Geometry check sheet. Reference: the model listing, model coordinates, mm. Give positions to 0.01 mm unless a question says otherwise; leave off trailing zeros. Loops run counter-clockwise (first coordinate to the right, second up) from the corner with the lowest first, then second, coordinate; pieces in that order, holes last. Notation, with made-up numbers: (84.25, 28.5) - (122.25, 28.5) arc R23 ccw to (122.25, 53.5) - close; hole circle Ø10 at (49.25, 28). An arc over 180 degrees is marked (long way). Use a Markdown table: item, result. Add a question column.
1. Cross-section at C-C on x = -27.35. Enter the section's corners in (y, z).
2. Material ranges on L1, parallel to Y at x = -61.55, z = 2.5; L2, parallel to X at y = 41.5, z = 4.5; L3, parallel to X at y = 43, z = 0.75, recorded low to high.
3. Depth check by flat-ended pin: P1, Ø5.5, axis at x = -27.35, y = 16.2, coming from the -Z side. Enter the tip coordinate at first touch or a pass-through.
4. Cross-section at A-A on y = 16.2. Enter the section's corners in (x, z), and give its area (3 significant figures).
5. Cross-section at B-B on x = -9.5. Enter the section's corners in (y, z), and give its area (3 significant figures).
6. Cross-section at D-D on z = 2.25. Enter the section's corners in (x, y) (3 decimals).
Autodesk Inventor part; units mm, degrees
ref_plane "YZ Plane" through (0, 0, 0) normal (1, 0, 0) x (0, 1, 0)
ref_plane "XZ Plane" through (0, 0, 0) normal (0, 1, 0) x (-1, 0, 0)
ref_plane "XY Plane" through (0, 0, 0) normal (0, 0, 1) x (1, 0, 0)
sketch "Sketch1" plane through (0, 0, 0) normal (0, 0, 1) x (1, 0, 0)
  line L0 (0, 0) -> (-88.9, 0)
  line L1 (-88.9, 0) -> (-88.9, 67.0052)
  line L2 (-88.9, 67.0052) -> (0, 67.0052)
  line L3 (0, 67.0052) -> (0, 0)
  dimension "d0" = 88.9
  dimension "d1" = 67.0052
  dimension "d2" = 90
extrude "Extrusion1" add sketch "Sketch1" along normal blind 6.35
sketch "Sketch2" plane through (-88.9, 67.0052, 0) normal (0, 1, 0) x (1, 0, 0)
  line L0 (0, 0) -> (88.9, 0)
  line L1 (0, 0) -> (0, -6.35)
  line L2 (88.9, -6.35) -> (0, -6.35)
  line L3 (88.9, 0) -> (88.9, -6.35)
sketch "Sketch3" plane through (0, 0, 0) normal (0, 0, -1) x (-1, 0, 0)
  line L0 (88.9, 0) -> (88.9, 67.0052)
  line L1 (0, 67.0052) -> (0, 0)
  line L2 (0, 67.0052) -> (0, 40.8178)
  line L3 (0, 40.8178) -> (6.35, 40.8178)
  line L4 (6.35, 40.8178) -> (6.35, 26.162)
  line L5 (6.35, 26.162) -> (12.7, 26.162)
  line L6 (12.7, 26.162) -> (12.7, 40.8178)
  line L7 (12.7, 40.8178) -> (6.35, 40.8178)
  line L8 (88.9, 40.8178) -> (82.55, 40.8178)
  line L9 (82.55, 40.8178) -> (82.55, 26.162)
  line L10 (82.55, 26.162) -> (76.2, 26.162)
  line L11 (76.2, 26.162) -> (76.2, 40.8178)
  line L12 (76.2, 40.8178) -> (82.55, 40.8178)
  dimension "d5" = 26.1874
  dimension "d6" = 6.35
  dimension "d7" = 14.6558
  dimension "d8" = 6.35
  dimension "d9" = 6.35
  dimension "d10" = 6.35
  dimension "d11" = 14.6558
extrude "Extrusion2" cut sketch "Sketch3" against normal blind 25.4
fillet "Fillet1" radius 3.175 4 edges at (0, 67.0052, 3.175) (0, 0, 3.175) (-88.9, 0, 3.175) (-88.9, 67.0052, 3.175)
sketch "Sketch4" plane through (0, 0, 0) normal (0, 0, -1) x (-1, 0, 0)
  circle A0 centre (61.55, 41.6) radius 3.3782
  circle A1 centre (61.55, 16.2) radius 3.3782
  circle A2 centre (27.35, 41.6) radius 3.3782
  circle A3 centre (27.35, 16.2) radius 3.3782
  point P0 (0, 0)
extrude "Extrusion3" cut sketch "Sketch4" against normal blind 25.4
properties part number "hook faceplate" material "Steel"
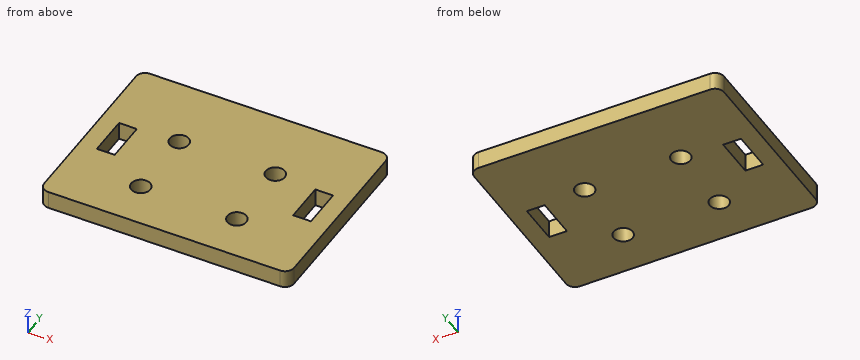
Values found:
| question | item | result |
|---|---|---|
| 1 | outline | (0, 0) - (12.82, 0) - (12.82, 6.35) - (0, 6.35) - close; (19.58, 0) - (38.22, 0) - (38.22, 6.35) - (19.58, 6.35) - close; (44.98, 0) - (67.01, 0) - (67.01, 6.35) - (44.98, 6.35) - close |
| 2 | L1 | y = 0 to 12.82, 19.58 to 38.22, 44.98 to 67.01 |
| 2 | L2 | x = -88.9 to -64.93, -58.17 to -30.73, -23.97 to 0 |
| 2 | L3 | x = -88.9 to -64.62, -58.48 to -30.42, -24.28 to 0 |
| 3 | P1 | passes through |
| 4 | outline | (-88.9, 0) - (-64.93, 0) - (-64.93, 6.35) - (-88.9, 6.35) - close; (-58.17, 0) - (-30.73, 0) - (-30.73, 6.35) - (-58.17, 6.35) - close; (-23.97, 0) - (0, 0) - (0, 6.35) - (-23.97, 6.35) - close |
| 4 | area | 479 mm2 |
| 5 | outline | (0, 0) - (26.16, 0) - (26.16, 6.35) - (0, 6.35) - close; (40.82, 0) - (67.01, 0) - (67.01, 6.35) - (40.82, 6.35) - close |
| 5 | area | 332 mm2 |
| 6 | outline | (-88.9, 3.175) arc R3.175 ccw to (-85.725, 0) - (-3.175, 0) arc R3.175 ccw to (0, 3.175) - (0, 63.83) arc R3.175 ccw to (-3.175, 67.005) - (-85.725, 67.005) arc R3.175 ccw to (-88.9, 63.83) - close; hole (-82.55, 26.162) - (-76.2, 26.162) - (-76.2, 40.818) - (-82.55, 40.818) - close; hole circle Ø6.756 at (-61.55, 16.2); hole circle Ø6.756 at (-61.55, 41.6); hole circle Ø6.756 at (-27.35, 16.2); hole circle Ø6.756 at (-27.35, 41.6); hole (-12.7, 26.162) - (-6.35, 26.162) - (-6.35, 40.818) - (-12.7, 40.818) - close |
